```python
from build123d import *

# Parameters (mm, degrees)
F1_DEPTH    = 90
F2_R        = 3
F3_T1_DEPTH = 113.3705433716


# Not quite as in the source:
# - a fillet or chamfer that OpenCascade refuses, or shapes differently, is made with other operations: its cross-section is extruded or revolved along the edge and cut away or added


with BuildPart() as f1:
    # F0 (on Top) → F1 (new body)
    with BuildSketch(Plane.XY):
        Polygon((-20, -17.5), (20, -17.5), (20, 12.5313148581), (-8.4129939735, -13.5), (-14.0197880107, -7.7935246759), (-14.2998851884, -3.8033435308), (-20, -10.4466760531), align=None)
    extrude(amount=F1_DEPTH)

    # F2
    f2_edges = [f1.edges().sort_by_distance(p)[0] for p in [
        (-20, -10.446676, 45),
        (20, 12.531315, 45),
    ]]
    fillet(f2_edges, radius=F2_R)

    # F3: fillet of radius 2 on 1 edges, made by hand

    # F3_s2 → F3_t1 (cut)
    with BuildSketch(Plane.XY.offset(-11.6852716858)):
        with BuildLine():
            ThreePointArc((-17.3435489028, -7.3506528059), (-15.5615402204, -6.6705242909), (-14.0197880107, -7.7935246759))
            Line((-14.0197880107, -7.7935246759), (-14.2998851884, -3.8033435308))
            Line((-14.2998851884, -3.8033435308), (-17.3435489028, -7.3506528059))
        make_face()
    extrude(amount=F3_T1_DEPTH, mode=Mode.SUBTRACT)


solid = f1.part
```
Part model, mm, in its own coordinate system. A direction names the side the tool comes from. Give positions to 0.01 mm unless a question says otherwise; leave off trailing zeros. Loops run counter-clockwise (first coordinate to the right, second up) from the corner with the lowest first, then second, coordinate; pieces in that order, holes last. Notation, with made-up numbers: M 24,-38.5 L 33,-38.5 A15 ccw 33,-24.5 Z; hole C 3,34 d7. An arc over 180 degrees is marked long. Return JSON: item names as keys, results as strings.
1) 3-axis set-ups, long thin cutter, end or side, ignore diameter. For faces 4 (the face through (-11.177, -10.687, 44.37)), 5 (the face through (0, -17.5, 44)): which of +Z, -Z, +X, -X, +Y, -Y reach the whole face in a straight line?
Calculated:
{"face 4": "+Z, -Z, +Y", "face 5": "+Z, -Z, +X, -X, -Y"}
2) Drill centre lines: line 1 (X direction, y = -13, z = 19); line 2 (X direction, y = -11.25, z = 13.5); line 3 (X direction, y = -2.75, z = 71). Where is each one in solid material? Low to high.
Calculated:
{"line 1": "x = -20 to -8.9, -7.87 to 20", "line 2": "x = -19.98 to -10.62, -5.96 to 20", "line 3": "x = 3.32 to 20"}
3) Pull direction X, two halves, no side cores. Call faces 1 (the face through (3.44, -2.64, 44.37)), 2 (the face through (4, -7, 0)), 3 (the face through (-20, -14, 44)): released by +X, released by -X, zero draft, split by the parting line, or undercut.
Calculated:
{"face 1": "undercut", "face 2": "zero draft", "face 3": "released by -X"}
4) Saw through at C-C, the plane y = -3.25. List the corners of the cut face in (x, z).
Calculated:
{"outline": "M 2.77,0 L 20,0 L 20,90 L 2.77,90 Z"}
5) Saw through at B-B, the plane x = 13. List the corners of the cut face in (y, z).
Calculated:
{"outline": "M -17.5,0 L 6.12,0 L 6.12,90 L -17.5,90 Z"}
6) Saw through at A-A, the plane z = 83.5. List the corners of the cut face in (x, y).
Calculated:
{"outline": "M -20,-17.5 L 20,-17.5 L 20,5.71 A3 ccw 14.97,7.93 L -8.41,-13.5 L -14.02,-7.79 A2 ccw -17.34,-7.35 L -19.28,-9.6 A3 ccw -20,-11.56 Z"}
7) Flat gauge pins, fed straight in: pin 1 Ø3 at (x, y) = (0, -3.5) entering from -Z; pin 2 Ø8 at (x, z) = (-12, 22.5) entering from +Y; pin 3 Ø1.5 at (x, z) = (-7.5, 29.5) entering from +Y. Where does each tip first touch, or does it go through?
Calculated:
{"pin 1": "passes through", "pin 2": "stops at y = -6.65", "pin 3": "stops at y = -11.98"}
